Build history of the part. All positions in model axes, mm. Face numbers are marked on the shaded views. A direction names the side the tool comes from. Give positions to 0.01 mm unless a question says otherwise; leave off trailing zeros. Order: outer loops, then holes, each group sorted by start corner. A loop starts at its lowest first (then second) coordinate and runs counter-clockwise, first axis right, second up. Notation, with made-up numbers: (-1.75, 52) - (21.25, 52) arc R16 ccw to (21.25, 58) - close; hole circle Ø2 at (66.5, 53). An arc over 180 degrees is marked (long way). Use a Markdown table: item, result.
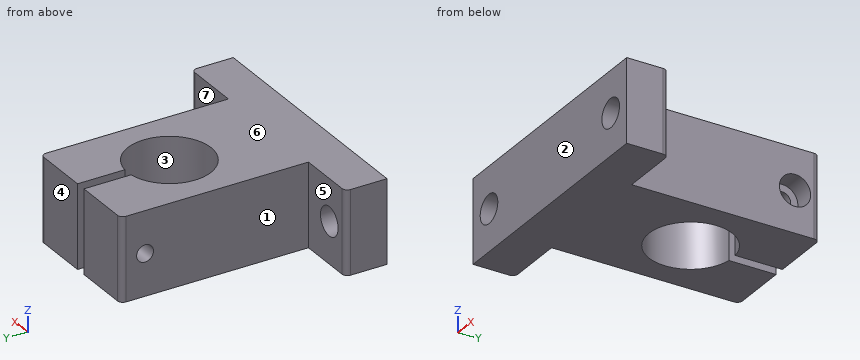
Autodesk Inventor part; units mm, degrees
ref_plane "YZ Plane" through (0, 0, 0) normal (1, 0, 0) x (0, 1, 0)
ref_plane "XZ Plane" through (0, 0, 0) normal (0, 1, 0) x (-1, 0, 0)
ref_plane "XY Plane" through (0, 0, 0) normal (0, 0, 1) x (1, 0, 0)
sketch "Esboço1" plane through (0, 0, 0) normal (0, 0, 1) x (1, 0, 0)
  line L0 (23.7277, -0.0451) -> (-24.2723, -0.0451)
  line L1 (-24.2723, -0.0451) -> (-24.2723, 7.9549)
  line L2 (23.7277, 7.9549) -> (23.7277, -0.0451)
  line L3 (12.2277, 43.9549) -> (12.2277, 7.9549)
  line L4 (-12.7723, 7.9549) -> (-12.7723, 43.9549)
  arc A0 (-1.2723, 34.8922) -> (0.7277, 34.8922) centre (-0.2723, 26.9549) ccw
  line L5 (-24.2723, 7.9549) -> (-12.7723, 7.9549)
  line L6 (12.2277, 7.9549) -> (23.7277, 7.9549)
  line L7 (0.7277, 43.9549) -> (0.7277, 34.8922)
  line L8 (-1.2723, 34.8922) -> (-1.2723, 43.9549)
  line L9 (-12.7723, 43.9549) -> (-1.2723, 43.9549)
  line L10 (0.7277, 43.9549) -> (12.2277, 43.9549)
  point P0 (-0.2723, 43.9549)
  dimension "largura" = 48
  dimension "largura_topo" = 25
  dimension "altura_base" = 8
  dimension "diametro" = 16
  dimension "altura_furo" = 27
  dimension "d6" = 11.5
  dimension "d7" = 12.5
  dimension "d8" = 8
  dimension "d10" = 11.5
  dimension "d11" = 11.5
extrude "Extrusão1" add sketch "Esboço1" along normal blind 16
sketch "Esboço2" plane through (12.2277, 7.9549, 0) normal (1, 0, 0) x (0, 0, -1)
  line L0 (0, 26.9373) -> (-16, 26.9373)
  line L1 (-8, 26.9373) -> (-8, 35.7534) construction
  circle A0 centre (-8, 31.3453) radius 1.1711 construction
  point P0 (0, -7.9549)
hole "Furo1" at (12.2277, 39.3003, 8) direction (-1, 0, 0) diameter 3.242 end through all counterbore diameter 6 counterbore depth 4
sketch "Esboço3" plane through (-24.2723, -0.0451, 0) normal (0, -1, 0) x (1, 0, 0)
  line L0 (5, 8) -> (43, 8) construction
  circle A0 centre (5, 8) radius 1 construction
  circle A1 centre (43, 8) radius 1 construction
  line L1 (48, 0) -> (0, 0) construction
  line L2 (24, 0) -> (24, 16) construction
  line L3 (0, 16) -> (48, 16) construction
  point P0 (24, 8)
  dimension "distancia_parafusos" = 38
  dimension "d22" = 2
  dimension "d23" = 2
hole "Furo2" at (-19.2723, -0.0451, 8) at (18.7277, -0.0451, 8) direction (0, 1, 0) diameter 5.5 end through all
fillet "Arredondamento1" radius 1 4 edges at (12.2277, 43.9549, 8) (-12.7723, 43.9549, 8) (-24.2723, 7.9549, 8) (23.7277, 7.9549, 8)
equation "\"d6\" = -0.5 * largura_topo + 0.5 * largura"
equation "\"d7\" = 0.5 * largura_topo"
equation "\"d8\" = altura_base"
equation "\"d11\" = d10"
properties part number "Sk16"
1) Slice it at B-B (y = 21). Write the cut outline in (x, z).
Computed:
| item | result |
|---|---|
| outline | (-12.77, 0) - (-5.61, 0) - (-5.61, 16) - (-12.77, 16) - close; (5.07, 0) - (12.23, 0) - (12.23, 16) - (5.07, 16) - close |
2) Two-plate mould, pull along Y, no slides. Class the marked faces 1, 2, 3 and 4: +Y half, -Y half, draft (parallel to the pull), parting line (faces both ways), or undercut.
Computed:
| item | result |
|---|---|
| face 1 | draft |
| face 2 | -Y half |
| face 3 | undercut |
| face 4 | +Y half |
3) Wall check: line 1 (X direction, y = 3.5, z = 8); line 2 (X direction, y = 27, z = 3); line 3 (Y direction, x = 5.5, z = 8). Give the ranges that are in metal, low to high. Write a range as from..to.
Computed:
| item | result |
|---|---|
| line 1 | x = -24.27..-22.02, -16.52..15.98, 21.48..23.73 |
| line 2 | x = -12.77..-8.27, 7.73..12.23 |
| line 3 | y = -0.05..21.42, 32.49..37.68, 40.92..43.95 |
4) Slice it at D-D (z = 1.5). Write the cut outline in (x, y).
Computed:
| item | result |
|---|---|
| outline | (-24.27, -0.05) - (23.73, -0.05) - (23.73, 6.95) arc R1 ccw to (22.73, 7.95) - (12.23, 7.95) - (12.23, 42.95) arc R1 ccw to (11.23, 43.95) - (0.73, 43.95) - (0.73, 34.89) arc R8 cw (long way) to (-1.27, 34.89) - (-1.27, 43.95) - (-11.77, 43.95) arc R1 ccw to (-12.77, 42.95) - (-12.77, 7.95) - (-23.27, 7.95) arc R1 ccw to (-24.27, 6.95) - close |
5) Tool access for the marked faces 5, 6 and 7: list every direction of +Z, -Z, +X, -X, +Y, -Y with a clear straight run to the whole face (end or side of a thin tool).
Computed:
| item | result |
|---|---|
| face 5 | +Z, -Z, -X, +Y |
| face 6 | +Z, +X, -X, +Y, -Y |
| face 7 | +Z, -Z, +X, +Y |
6) Slice it at C-C (z = 8). State how many separate pieces and enclosed holes the cut face has, and give its area (3 significant figures).
Computed:
| item | result |
|---|---|
| separate pieces | 5 |
| enclosed holes | 0 |
| area | 890 mm² |
7) Pin check, flat tips, straight feed: P1, Ø3.5, axis at y = 39.3, z = 8, coming from the +X side; P2, Ø6.5, axis at y = 38, z = 8.5, coming from the +X side; P3, Ø8.5, axis at x = 18.5, z = 8.5, coming from the +Y side. Stop position of each tip, or through.
Computed:
| item | result |
|---|---|
| P1 | stops at x = 8.23 |
| P2 | stops at x = 12.23 |
| P3 | stops at y = 7.95 |
8) Slice it at A-A (x = 6). Write the cut outline in (y, z), and give its area (3 significant figures).
Computed:
| item | result |
|---|---|
| outline | (-0.05, 0) - (21.99, 0) - (21.99, 16) - (-0.05, 16) - close; (31.92, 0) - (43.95, 0) - (43.95, 16) - (31.92, 16) - close; hole circle Ø3.24 at (39.3, 8) |
| area | 537 mm² |
